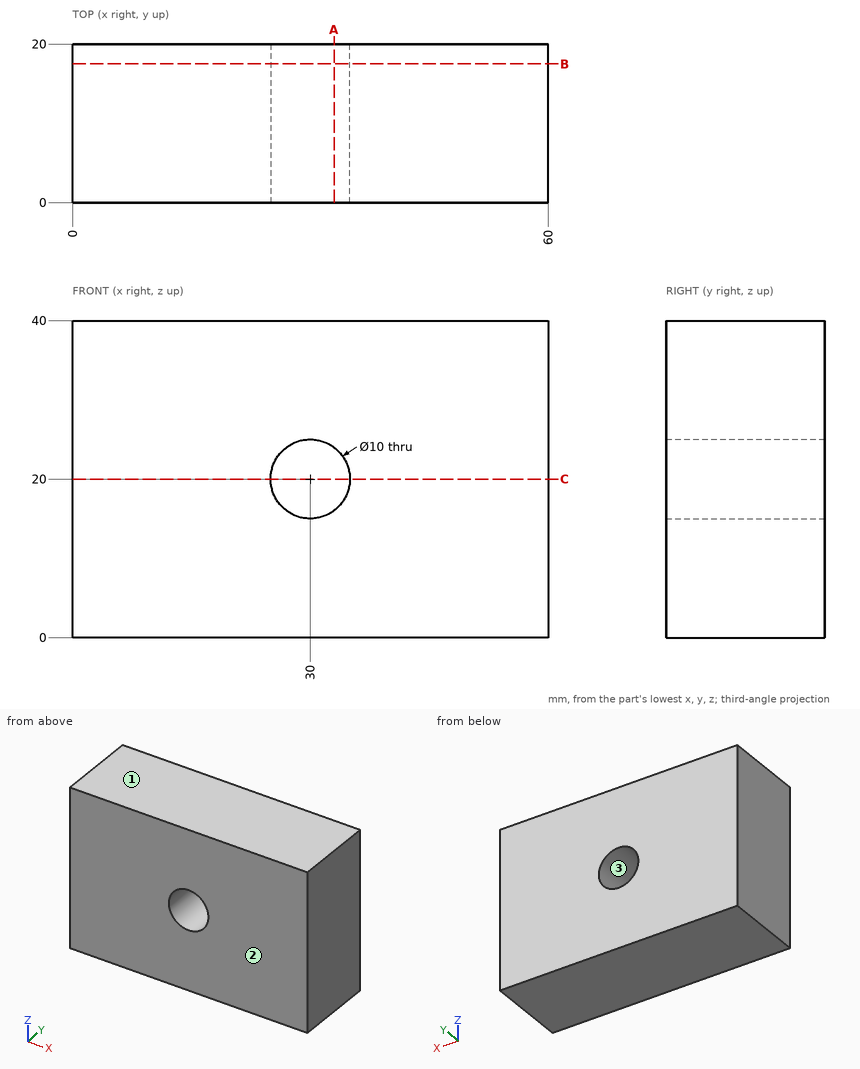
The drawing under review shows one solid part. Ordinate dimensions are in mm from its lowest x, y, z. Round coordinates to 2 decimals unless told otherwise and drop trailing zeros. Write each loop counter-clockwise with the first axis right and the second up, starting at its lowest first coordinate (ties: lowest second). Pieces come first, ordered by that corner, then holes. Notation, with made-up numbers: (70.25, 18.25) - (84.25, 18.25) arc R13 ccw to (84.25, 41.25) - close; hole circle Ø4 at (-10.5, 81.5). An arc over 180 degrees is marked (long way). Use a Markdown table: item, result. Add a question column.
1. We need section B-B (y = 17.5). State the section outline as (x, z) points.
2. Mouldability with a two-part tool opening along Z and no side actions: class the marked faces 1, 2 and 3 as +Z half, -Z half, draft (parallel to the pull), parting line (faces both ways), or undercut.
3. We need section A-A (x = 33). State the section outline as (y, z) points.
4. Wall thickness on probe 1 along Z at (x, y) = (30, 12.5); probe 2 along X at (y, z) = (10.25, 21): over which ranges is each line inside the solid? List them lowest first.
5. We need section C-C (z = 20). State the section outline as (x, y) points.
Output:
| question | item | result |
|---|---|---|
| 1 | outline | (0, 0) - (60, 0) - (60, 40) - (0, 40) - close; hole circle Ø10 at (30, 20) |
| 2 | face 1 | +Z half |
| 2 | face 2 | draft |
| 2 | face 3 | undercut |
| 3 | outline | (0, 0) - (20, 0) - (20, 16) - (0, 16) - close; (0, 24) - (20, 24) - (20, 40) - (0, 40) - close |
| 4 | probe 1 | z = 0 to 15, 25 to 40 |
| 4 | probe 2 | x = 0 to 25.1, 34.9 to 60 |
| 5 | outline | (0, 0) - (25, 0) - (25, 20) - (0, 20) - close; (35, 0) - (60, 0) - (60, 20) - (35, 20) - close |
